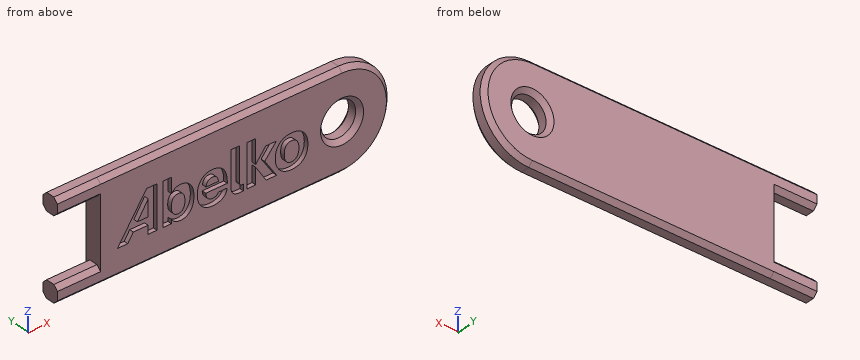
```python
from build123d import *

# Parameters (mm, degrees)
F0_R     = 2
F1_DEPTH = 2
F3_DEPTH = 0.5
F6_DEPTH = 5
F7_SIZE  = 0.49999


# Not quite as in the source:
# - a fillet or chamfer is up to 0.001 mm smaller than in the source, because OpenCascade refuses the exact size
# - a feature names something its author has since deleted; it is built from what else it names


with BuildPart() as f1:
    # F0 (on Front) → F1 (new body)
    with BuildSketch(Plane.XZ):
        with BuildLine():
            Line((-18, 5.15), (-13, 5.15))
            Line((-13, 5.15), (-13, -2.15))
            Line((-13, -2.15), (-18, -2.15))
            Line((-18, -2.15), (-18, -4.15))
            Line((-18, -4.15), (15, -4.15))
            ThreePointArc((15, -4.15), (20.65, 1.5), (15, 7.15))
            Line((15, 7.15), (-18, 7.15))
            Line((-18, 7.15), (-18, 5.15))
        make_face()
        with Locations((15, 1.5)):
            Circle(F0_R, mode=Mode.SUBTRACT)
    extrude(amount=F1_DEPTH)

    # F2 (on face) → F3 (cut)
    with BuildSketch(Plane.XZ.offset(2)):
        Polygon((-6.4611563108, -1.0079550547), (-6.4611104663, 3.943059476), (-7.6544608052, 3.943059476), (-11.0437756499, -1.0079550547), (-9.8374226558, -1.0079550547), (-9.200951568, -0.0383489504), (-7.4783776914, -0.0383489504), (-7.4783776914, -1.0079550547), align=None)
        Polygon((-7.4783776914, 0.8486796922), (-8.7143920972, 0.8486796922), (-7.4783776914, 2.7703563678), align=None, mode=Mode.SUBTRACT)
        with BuildLine():
            add(Edge.make_bspline(
                [(-4.7631894864, 2.1669850315), (-4.5225056976, 2.5245150692), (-4.1993017526, 2.7308727653), (-3.7111148009, 2.7308727653)],
                knots=[0, 0, 0, 0, 1, 1, 1, 1], degree=3))
            Line((-4.7631894864, 2.1669850315), (-4.7631894864, 3.927357724))
            Line((-4.7631894864, 3.927357724), (-5.7603080401, 3.927357724))
            Line((-5.7603080401, 3.927357724), (-5.7603080401, -1.0167973187))
            Line((-5.7603080401, -1.0167973187), (-4.7838195254, -1.0167973187))
            Line((-4.7838195254, -1.0167973187), (-4.7838195254, -0.5561170858))
            add(Edge.make_bspline(
                [(-3.6973614416, -1.1130536425), (-4.1993017526, -1.1130536425), (-4.4812456195, -0.9686490998), (-4.7838195254, -0.5561170858)],
                knots=[0, 0, 0, 0, 1, 1, 1, 1], degree=3))
            add(Edge.make_bspline(
                [(-2.1707958582, 0.8604731979), (-2.1707958582, -0.4666858665), (-2.8515298409, -1.1130536425), (-3.6973614416, -1.1130536425)],
                knots=[0, 0, 0, 0, 1, 1, 1, 1], degree=3))
            add(Edge.make_bspline(
                [(-3.7111148009, 2.7308727653), (-2.8171464425, 2.7308727653), (-2.1707958582, 2.0363281176), (-2.1707958582, 0.8604731979)],
                knots=[0, 0, 0, 0, 1, 1, 1, 1], degree=3))
        make_face()
        with BuildLine():
            add(Edge.make_bspline(
                [(-3.9724286288, -0.2947688745), (-3.5529511683, -0.2947688745), (-3.2159938639, 0.0352945585), (-3.2159938639, 0.7504520535)],
                knots=[0, 0, 0, 0, 1, 1, 1, 1], degree=3))
            add(Edge.make_bspline(
                [(-4.7975728848, 0.7573230027), (-4.7975728848, 0.1109609572), (-4.4881796048, -0.2947688745), (-3.9724286288, -0.2947688745)],
                knots=[0, 0, 0, 0, 1, 1, 1, 1], degree=3))
            add(Edge.make_bspline(
                [(-4.0067547215, 1.8575344459), (-4.5362590569, 1.8575344459), (-4.7975728848, 1.4518218059), (-4.7975728848, 0.7573230027)],
                knots=[0, 0, 0, 0, 1, 1, 1, 1], degree=3))
            add(Edge.make_bspline(
                [(-3.2159938639, 0.7504520535), (-3.2159938639, 1.5275053963), (-3.4910610511, 1.8575344459), (-4.0067547215, 1.8575344459)],
                knots=[0, 0, 0, 0, 1, 1, 1, 1], degree=3))
        make_face(mode=Mode.SUBTRACT)
        with BuildLine():
            add(Edge.make_bspline(
                [(-0.0526639052, 2.744568819), (1.0544242177, 2.744568819), (1.7351582004, 2.0775881956), (1.6938981223, 0.5441058186)],
                knots=[0, 0, 0, 0, 1, 1, 1, 1], degree=3))
            add(Edge.make_bspline(
                [(-1.785529879, 0.7848583742), (-1.785529879, 2.0156980785), (-1.0566591386, 2.744568819), (-0.0526639052, 2.744568819)],
                knots=[0, 0, 0, 0, 1, 1, 1, 1], degree=3))
            add(Edge.make_bspline(
                [(0.0092262119, -1.1405660918), (-0.8434820685, -1.1405660918), (-1.785529879, -0.6386028585), (-1.785529879, 0.7848583742)],
                knots=[0, 0, 0, 0, 1, 1, 1, 1], degree=3))
            add(Edge.make_bspline(
                [(1.6870214426, 0.0421253936), (1.6251313255, -0.5973026665), (1.0337941786, -1.1405660918), (0.0092262119, -1.1405660918)],
                knots=[0, 0, 0, 0, 1, 1, 1, 1], degree=3))
            Line((1.6870214426, 0.0421253936), (0.6624534759, 0.0421253936))
            add(Edge.make_bspline(
                [(0.0160455859, -0.3360690666), (0.2705400398, -0.3360690666), (0.5455499213, -0.2466435779), (0.6624534759, 0.0421253936)],
                knots=[0, 0, 0, 0, 1, 1, 1, 1], degree=3))
            add(Edge.make_bspline(
                [(-0.7953453107, 0.5441058186), (-0.788468631, 0.0352945585), (-0.5202781235, -0.3360690666), (0.0160455859, -0.3360690666)],
                knots=[0, 0, 0, 0, 1, 1, 1, 1], degree=3))
            Line((-0.7953453107, 0.5441058186), (1.6938981223, 0.5441058186))
        make_face()
        with BuildLine():
            add(Edge.make_bspline(
                [(0.6693301556, 1.1905423614), (0.6487001165, 1.6443344535), (0.4011969537, 1.933235228), (-0.0457872255, 1.933235228)],
                knots=[0, 0, 0, 0, 1, 1, 1, 1], degree=3))
            Line((0.6693301556, 1.1905423614), (-0.767838592, 1.1905423614))
            add(Edge.make_bspline(
                [(-0.0457872255, 1.933235228), (-0.4652646861, 1.933235228), (-0.7059484749, 1.6512741694), (-0.767838592, 1.1905423614)],
                knots=[0, 0, 0, 0, 1, 1, 1, 1], degree=3))
        make_face(mode=Mode.SUBTRACT)
        with BuildLine():
            add(Edge.make_bspline(
                [(3.3833837085, -0.3222813238), (3.4383971459, -0.3222813238), (3.5277366761, -0.3222813238), (3.5689967542, -0.3153416079)],
                knots=[0, 0, 0, 0, 1, 1, 1, 1], degree=3))
            add(Edge.make_bspline(
                [(3.1151358953, 0.0215526602), (3.1151358953, -0.2122831017), (3.2183433962, -0.3222813238), (3.3833837085, -0.3222813238)],
                knots=[0, 0, 0, 0, 1, 1, 1, 1], degree=3))
            Line((3.1151358953, 0.0215526602), (3.1151358953, 3.9342344037))
            Line((3.1151358953, 3.9342344037), (2.1249513269, 3.9342344037))
            Line((2.1249513269, 3.9342344037), (2.1249513269, -0.1228518825))
            add(Edge.make_bspline(
                [(3.1151358953, -1.0649283459), (2.3656351158, -1.0649283459), (2.1249513269, -0.6180129335), (2.1249513269, -0.1228518825)],
                knots=[0, 0, 0, 0, 1, 1, 1, 1], degree=3))
            add(Edge.make_bspline(
                [(3.5689967542, -1.0580975107), (3.4177098012, -1.0649283459), (3.2664801539, -1.0649283459), (3.1151358953, -1.0649283459)],
                knots=[0, 0, 0, 0, 1, 1, 1, 1], degree=3))
            Line((3.5689967542, -1.0580975107), (3.5689967542, -0.3153416079))
        make_face()
        Polygon((4.9878276893, 1.1561131185), (4.9878276893, 3.9136043647), (4.0113964803, 3.9136043647), (4.0113964803, -1.0167973187), (4.9878276893, -1.0167973187), (4.9878276893, 0.8673498775), (6.1980660074, -1.0167973187), (7.4220576849, -1.0167973187), (6.0399023747, 1.0392668696), (7.3739782328, 2.6345419441), (6.1499292496, 2.6345419441), align=None)
        with BuildLine():
            add(Edge.make_bspline(
                [(9.1528033491, 2.7652561637), (10.3630416672, 2.7652561637), (11.0437756499, 2.0088213988), (11.0437756499, 0.7985830807)],
                knots=[0, 0, 0, 0, 1, 1, 1, 1], degree=3))
            add(Edge.make_bspline(
                [(7.2617737426, 0.8122791344), (7.2617737426, 1.940054602), (7.928754366, 2.7652561637), (9.1528033491, 2.7652561637)],
                knots=[0, 0, 0, 0, 1, 1, 1, 1], degree=3))
            add(Edge.make_bspline(
                [(9.1596800288, -1.1474141187), (7.9700144441, -1.1474141187), (7.2617737426, -0.3497708508), (7.2617737426, 0.8122791344)],
                knots=[0, 0, 0, 0, 1, 1, 1, 1], degree=3))
            add(Edge.make_bspline(
                [(11.0437756499, 0.7985830807), (11.0437756499, -0.3222813238), (10.4042444396, -1.1474141187), (9.1596800288, -1.1474141187)],
                knots=[0, 0, 0, 0, 1, 1, 1, 1], degree=3))
        make_face()
        with BuildLine():
            add(Edge.make_bspline(
                [(9.1528033491, -0.3153416079), (9.6753736992, -0.3153416079), (10.0053970182, 0.090319457), (10.0053970182, 0.7985830807)],
                knots=[0, 0, 0, 0, 1, 1, 1, 1], degree=3))
            add(Edge.make_bspline(
                [(8.3000950687, 0.8122791344), (8.3000950687, 0.0628528523), (8.6163650284, -0.3153416079), (9.1528033491, -0.3153416079)],
                knots=[0, 0, 0, 0, 1, 1, 1, 1], degree=3))
            add(Edge.make_bspline(
                [(9.1528033491, 1.933235228), (8.7539559276, 1.933235228), (8.3000950687, 1.7337599422), (8.3000950687, 0.8122791344)],
                knots=[0, 0, 0, 0, 1, 1, 1, 1], degree=3))
            add(Edge.make_bspline(
                [(10.0053970182, 0.7985830807), (10.0053970182, 1.5618429502), (9.6615630342, 1.933235228), (9.1528033491, 1.933235228)],
                knots=[0, 0, 0, 0, 1, 1, 1, 1], degree=3))
        make_face(mode=Mode.SUBTRACT)
    extrude(amount=-F3_DEPTH, mode=Mode.SUBTRACT)

    # F4 (on face) + F5 (on face) → F6 (cut)
    with BuildSketch(Plane(origin=(-18, 0, 0), x_dir=(0, -1, 0), z_dir=(-1, 0, 0))):
        Polygon((0.5, 5.15), (0, 5.65), (0, 5.15), align=None)
        Polygon((0, 7.15), (0, 6.65), (0.5, 7.15), align=None)
        Polygon((2, 7.15), (1.5, 7.15), (2, 6.65), align=None)
        Polygon((2, 5.65), (1.5, 5.15), (2, 5.15), align=None)
    with BuildSketch(Plane(origin=(-18, 0, 0), x_dir=(0, -1, 0), z_dir=(-1, 0, 0))):
        Polygon((0, -2.15), (0, -2.65), (0.5, -2.15), align=None)
        Polygon((2, -2.15), (1.5, -2.15), (2, -2.65), align=None)
        Polygon((2, -3.65), (1.5, -4.15), (2, -4.15), align=None)
        Polygon((0.5, -4.15), (0, -3.65), (0, -4.15), align=None)
    extrude(amount=-F6_DEPTH, mode=Mode.SUBTRACT)

    # F7 (size 0.5 in the source; OpenCascade refuses exactly that, so slightly less here)
    f7_edges = [f1.edges().sort_by_distance(p)[0] for p in [
        (1, -2, -4.15),
        (20.65, -2, 1.5),
        (1, -2, 7.15),
        (1, 0, -4.15),
        (13, -2, 1.5),
        (13, 0, 1.5),
    ]]
    chamfer(f7_edges, length=F7_SIZE)


solid = f1.part
```
For this review, take the finished solid that the model builds, in its own axes (mm). Round coordinates to 2 decimals unless told otherwise and drop trailing zeros. Write each loop counter-clockwise with the first axis right and the second up, starting at its lowest first coordinate (ties: lowest second). Pieces come first, ordered by that corner, then holes. Notation, with made-up numbers: (29.25, 86.25) -> (82.25, 86.25) arc R18 ccw to (82.25, 108.25) -> close; hole circle Ø5 at (70.25, 70.25). An arc over 180 degrees is marked (long way). Use one line per item in the form item = value.
1) Take a section at A-A, the plane y = -1.15. Write out the cut boundary in (x, z), and give its area (3 significant figures).
Found:
outline = (-18, -4.15) -> (15, -4.15) arc R5.65 ccw to (15, 7.15) -> (-18, 7.15) -> (-18, 5.15) -> (-13, 5.15) -> (-13, -2.15) -> (-18, -2.15) -> close; hole circle Ø4 at (15, 1.5)
area = 374 mm2
2) Clearance check with flat-ended pins moving along their axes: pin 1 (2.5 mm diameter, centred on x = 15, z = 1.5, fed in from +Y); pin 2 (0.6 mm diameter, centred on x = -10.5, y = -2, fed in from +Z); pin 3 (4 mm diameter, centred on x = 6, z = 2, fed in from -Y); pin 4 (0.6 mm diameter, centred on y = -2, z = -0.5, fed in from -X). State where each tip first meets the part, or that it passes through.
Found:
pin_1 = through
pin_2 = 6.95
pin_3 = -2
pin_4 = -13
3) To check wall thickness, follow L1, parallel to Z at x = 9, y = -1.6; L2, parallel to X at y = -0.35, z = 0.5; L3, parallel to X at y = -0.8, z = 3. State the ranges of each line that lie inside material, in increasing order. Write a range as from..to.
Found:
L1 = -4.05..-1.14, -0.3..1.92, 2.76..7.05
L2 = -13..13.1, 16.9..20.41
L3 = -13..13.68, 16.32..20.45
